Part model, mm, in its own coordinate system. A direction names the side the tool comes from. Coordinates: 2 decimals unless noted, no trailing zeros. Write each loop counter-clockwise with the first axis right and the second up, starting at its lowest first coordinate (ties: lowest second). Pieces come first, ordered by that corner, then holes. Notation, with made-up numbers: (32, 65) - (47, 65) arc R10 ccw to (47, 84) - close; hole circle Ø4 at (69, 12.5). An arc over 180 degrees is marked (long way). Write each question's results on one line, items separated by ' | '.
from build123d import *

# Parameters (mm, degrees)
SKETCH2_R           = 3.95
BOSS_EXTRUDE1_DEPTH = 13.25
SKETCH3_R           = 8.25
BOSS_EXTRUDE2_DEPTH = 6.25
CUT_EXTRUDE1_DEPTH  = 4
BOSS_EXTRUDE3_DEPTH = 6.25


with BuildPart() as part:
    # Sketch2 → Boss-Extrude1 (new body)
    with BuildSketch(Plane(origin=(0, 0, 0), x_dir=(1, 0, 0), z_dir=(0, 1, 0))):
        with Locations(Location((0, 0, 0), (0, 0, 270))):
            Circle(SKETCH2_R)
    extrude(amount=BOSS_EXTRUDE1_DEPTH)

    # Sketch3 → Boss-Extrude2 (add)
    with BuildSketch(Plane(origin=(0, 13.25, 0), x_dir=(1, 0, 0), z_dir=(0, 1, 0))):
        with Locations(Location((0, 0, 0), (0, 0, 270))):
            Circle(SKETCH3_R)
    extrude(amount=-BOSS_EXTRUDE2_DEPTH)

    # Sketch5 → Cut-Extrude1 (cut)
    with BuildSketch(Plane(origin=(0, 13.25, 0), x_dir=(1, 0, 0), z_dir=(0, 1, 0))):
        with BuildLine():
            Line((0.25, -0.968245837), (0.25, -1.5))
            Line((0.25, -1.5), (-0.25, -1.5))
            Line((-0.25, -1.5), (-0.25, -0.968245837))
            ThreePointArc((-0.25, -0.968245837), (-1, 0), (-0.25, 0.968245837))
            Line((-0.25, 0.968245837), (-0.25, 1.5))
            Line((-0.25, 1.5), (0.25, 1.5))
            Line((0.25, 1.5), (0.25, 0.968245837))
            ThreePointArc((0.25, 0.968245837), (1, 0), (0.25, -0.968245837))
        make_face()
    extrude(amount=-CUT_EXTRUDE1_DEPTH, mode=Mode.SUBTRACT)

    # Sketch4 → Boss-Extrude3 (add)
    with BuildSketch(Plane(origin=(0, 7, 0), x_dir=(1, 0, 0), z_dir=(0, 1, 0))):
        with BuildLine():
            Line((0, 8.25), (-1.301452207, 11.545140545))
            ThreePointArc((-1.301452207, 11.545140545), (0.465666366, 9.883034259), (2, 8.003905297))
            Line((2, 8.003905297), (0, 8.25))
        make_face()
        with BuildLine():
            Line((2.821666182, 7.752464121), (2.725705589, 11.294006247))
            ThreePointArc((2.725705589, 11.294006247), (3.817780042, 9.127747087), (4.616882078, 6.837170458))
            Line((4.616882078, 6.837170458), (2.821666182, 7.752464121))
        make_face()
        with BuildLine():
            Line((5.30299778, 6.319866656), (6.424103064, 9.680648113))
            ThreePointArc((6.424103064, 9.680648113), (6.7094131, 7.271518905), (6.67690004, 4.845771956))
            Line((6.67690004, 4.845771956), (5.30299778, 6.319866656))
        make_face()
        with BuildLine():
            Line((7.144709581, 4.125), (9.347658899, 6.899660946))
            ThreePointArc((9.347658899, 6.899660946), (8.791791918, 4.538238227), (7.931585317, 2.269901841))
            Line((7.931585317, 2.269901841), (7.144709581, 4.125))
        make_face()
        with BuildLine():
            Line((8.124663962, 1.432597466), (11.143749115, 3.28647284))
            ThreePointArc((11.143749115, 3.28647284), (9.813750878, 1.257579041), (8.229604346, -0.579751937))
            Line((8.229604346, -0.579751937), (8.124663962, 1.432597466))
        make_face()
        with BuildLine():
            Line((8.124663962, -1.432597466), (11.595738723, -0.723112393))
            ThreePointArc((11.595738723, -0.723112393), (9.652026646, -2.174762737), (7.535011635, -3.359479075))
            Line((7.535011635, -3.359479075), (8.124663962, -1.432597466))
        make_face()
        with BuildLine():
            Line((7.144709581, -4.125), (10.649111106, -4.6454796))
            ThreePointArc((10.649111106, -4.6454796), (8.326125552, -5.344796032), (5.931585317, -5.734003456))
            Line((5.931585317, -5.734003456), (7.144709581, -4.125))
        make_face()
        with BuildLine():
            Line((5.30299778, -6.319866656), (8.418043526, -8.007533407))
            ThreePointArc((8.418043526, -8.007533407), (5.995970836, -7.870168046), (3.612722268, -7.416922395))
            Line((3.612722268, -7.416922395), (5.30299778, -6.319866656))
        make_face()
        with BuildLine():
            Line((2.821666182, -7.752464121), (5.171635659, -10.403760506))
            ThreePointArc((5.171635659, -10.403760506), (2.942613546, -9.446281642), (0.858111595, -8.205251032))
            Line((0.858111595, -8.205251032), (2.821666182, -7.752464121))
        make_face()
        with BuildLine():
            Line((0, -8.25), (1.301452207, -11.545140545))
            ThreePointArc((1.301452207, -11.545140545), (-0.465666366, -9.883034259), (-2, -8.003905297))
            Line((-2, -8.003905297), (0, -8.25))
        make_face()
        with BuildLine():
            Line((-2.821666182, -7.752464121), (-2.725705589, -11.294006247))
            ThreePointArc((-2.725705589, -11.294006247), (-3.817780042, -9.127747087), (-4.616882078, -6.837170458))
            Line((-4.616882078, -6.837170458), (-2.821666182, -7.752464121))
        make_face()
        with BuildLine():
            Line((-5.30299778, -6.319866656), (-6.424103064, -9.680648113))
            ThreePointArc((-6.424103064, -9.680648113), (-6.7094131, -7.271518905), (-6.67690004, -4.845771956))
            Line((-6.67690004, -4.845771956), (-5.30299778, -6.319866656))
        make_face()
        with BuildLine():
            Line((-7.144709581, -4.125), (-9.347658899, -6.899660946))
            ThreePointArc((-9.347658899, -6.899660946), (-8.791791918, -4.538238227), (-7.931585317, -2.269901841))
            Line((-7.931585317, -2.269901841), (-7.144709581, -4.125))
        make_face()
        with BuildLine():
            Line((-8.124663962, -1.432597466), (-11.143749115, -3.28647284))
            ThreePointArc((-11.143749115, -3.28647284), (-9.813750878, -1.257579041), (-8.229604346, 0.579751937))
            Line((-8.229604346, 0.579751937), (-8.124663962, -1.432597466))
        make_face()
        with BuildLine():
            Line((-8.124663962, 1.432597466), (-11.595738723, 0.723112393))
            ThreePointArc((-11.595738723, 0.723112393), (-9.652026646, 2.174762737), (-7.535011635, 3.359479075))
            Line((-7.535011635, 3.359479075), (-8.124663962, 1.432597466))
        make_face()
        with BuildLine():
            Line((-7.144709581, 4.125), (-10.649111106, 4.6454796))
            ThreePointArc((-10.649111106, 4.6454796), (-8.326125552, 5.344796032), (-5.931585317, 5.734003456))
            Line((-5.931585317, 5.734003456), (-7.144709581, 4.125))
        make_face()
        with BuildLine():
            Line((-5.30299778, 6.319866656), (-8.418043526, 8.007533407))
            ThreePointArc((-8.418043526, 8.007533407), (-5.995970836, 7.870168046), (-3.612722268, 7.416922395))
            Line((-3.612722268, 7.416922395), (-5.30299778, 6.319866656))
        make_face()
        with BuildLine():
            Line((-2.821666182, 7.752464121), (-5.171635659, 10.403760506))
            ThreePointArc((-5.171635659, 10.403760506), (-2.942613546, 9.446281642), (-0.858111595, 8.205251032))
            Line((-0.858111595, 8.205251032), (-2.821666182, 7.752464121))
        make_face()
    extrude(amount=BOSS_EXTRUDE3_DEPTH)


solid = part.part
(1) Saw through at B-B on z = 0. Write the cut outline in (x, y), then the cut area to 3 significant figures.
Return value:
outline: (-8.78, 7) - (-3.95, 7) - (-3.95, 0) - (3.95, 0) - (3.95, 7) - (8.78, 7) - (8.78, 13.25) - (1, 13.25) - (1, 9.25) - (-1, 9.25) - (-1, 13.25) - (-8.78, 13.25) - close | area: 157 mm^2
(2) Saw through at C-C on y = 6.5. Write the cut outline in (x, z), then the cut area to 3 significant figures.
Return value:
outline: circle Ø7.9 at (0, 0) | area: 49.0 mm^2
(3) Two-plate mould, pull along Z, no slides. Class faces 1 (the flat face through (-5.856, 10.081, 7.977)), 2 (the cylindrical face through (3.804, 10.081, -9.159)), 3 (the cylindrical face through (0.42, 10.17, 8.24)): released by +Z, released by -Z, zero draft, split by the parting line, or undercut.
Return value:
face 1: released by +Z | face 2: released by -Z | face 3: undercut
(4) 3-axis set-ups, long thin cutter, end or side, ignore diameter. For faces 4 (the flat face through (-0.64, 10.08, -9.87)), 5 (the cylindrical face through (0.44, 10.08, -9.91)), 6 (the cylindrical face through (-8.359, 10.081, -5.337)): which of +Z, -Z, +X, -X, +Y, -Y reach the whole face in a straight line?
Return value:
face 4: +Y, -Y | face 5: -Z, +Y, -Y | face 6: -X, +Y, -Y
(5) Flat gauge pins, fed straight in: P1, Ø12, axis at x = -8, z = 7.5, coming from the -Y side; P2, Ø0.6, axis at x = 0.5, z = 0, coming from the +Y side; P3, Ø4, axis at y = 7.5, z = -6.5, coming from the +X side. Where does each tip first touch, or does it go through?
Return value:
P1: stops at y = 7 | P2: stops at y = 9.25 | P3: stops at x = 9.35
(6) Wall check: line 1 (Z direction, x = 10, y = 7.25); line 2 (Y direction, x = -3.5, z = -4); line 3 (Z direction, x = 3, y = 10.5). Give the ranges that are in metal, low to high. Write a range as from..to.
Return value:
line 1: z = -2.58..-1.51, 1.05..1.94, 4.55..4.87 | line 2: y = 7..13.25 | line 3: z = -10.81..7.69, 7.95..9.48
(7) Saw through at A-A on x = -9.75. Write the cut outline in (y, z).
Return value:
outline: (7, -4.96) - (13.25, -4.96) - (13.25, -4.51) - (7, -4.51) - close; (7, -2.11) - (13.25, -2.11) - (13.25, -1.1) - (7, -1.1) - close; (7, 1.17) - (13.25, 1.17) - (13.25, 2.43) - (7, 2.43) - close
